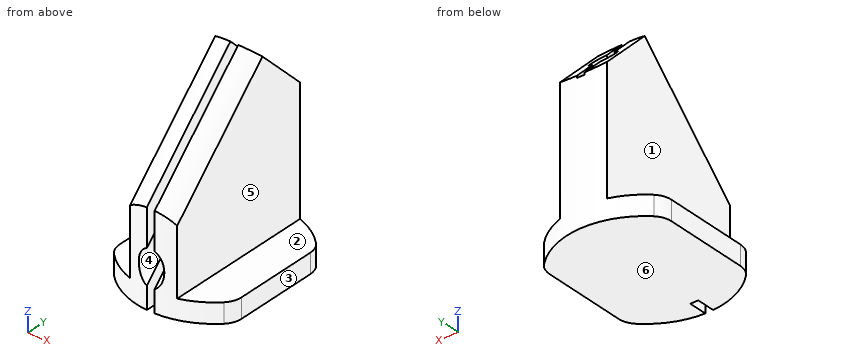
from build123d import *

# Parameters (mm, degrees)
BOSS_EXTRUDE1_DEPTH     = 50
CUT_EXTRUDE2_DEPTH      = 21
CUT_EXTRUDE2_DEPTH_BACK = 21
CUT_EXTRUDE3_DEPTH      = 10.5
CUT_EXTRUDE3_DEPTH_BACK = 22.5
CUT_EXTRUDE4_DEPTH      = 54.639610307


with BuildPart() as part:
    # Sketch1 → Boss-Extrude1 (new body)
    with BuildSketch(Plane.XY):
        with BuildLine():
            Line((-15.5, 10.712142643), (-15.5, -10.712142643))
            ThreePointArc((-15.5, -10.712142643), (-15.109772229, -12.648634316), (-14, -14.282856857))
            ThreePointArc((-14, -14.282856857), (0, -20), (14, -14.282856857))
            ThreePointArc((14, -14.282856857), (15.109772229, -12.648634316), (15.5, -10.712142643))
            Line((15.5, -10.712142643), (15.5, 10.712142643))
            ThreePointArc((15.5, 10.712142643), (15.109772229, 12.648634316), (14, 14.282856857))
            ThreePointArc((14, 14.282856857), (0, 20), (-14, 14.282856857))
            ThreePointArc((-14, 14.282856857), (-15.109772229, 12.648634316), (-15.5, 10.712142643))
        make_face()
    extrude(amount=BOSS_EXTRUDE1_DEPTH)

    # Sketch3 → Cut-Extrude2 (cut, two sides)
    with BuildSketch(Plane(origin=(0, 0, 0), x_dir=(1, 0, 0), z_dir=(0, 1, 0))) as cut_extrude2_sk:
        Polygon((-142.514750581, -5), (-18.067603989, -5), (-6, -5), (-6, -53.756778028), (6, -53.756778028), (6, -5), (19.848795464, -5), (144.295942056, -5), (144.295942056, -253.894293184), (-142.514750581, -253.894293184), align=None)
    extrude(amount=CUT_EXTRUDE2_DEPTH, mode=Mode.SUBTRACT)
    extrude(cut_extrude2_sk.sketch, amount=-CUT_EXTRUDE2_DEPTH_BACK, mode=Mode.SUBTRACT)

    # Sketch4 → Cut-Extrude3 (cut, two sides)
    with BuildSketch(Plane.ZY.offset(6)) as cut_extrude3_sk:
        Polygon((143.928068638, -88.070204261), (54.263494486, 1.594369891), (31.585867619, 24.271996758), (-58.078706533, 113.93657091), (121.250441771, 293.265719213), (323.257216942, 91.258944042), align=None)
    extrude(amount=CUT_EXTRUDE3_DEPTH, mode=Mode.SUBTRACT)
    extrude(cut_extrude3_sk.sketch, amount=-CUT_EXTRUDE3_DEPTH_BACK, mode=Mode.SUBTRACT)

    # Sketch5 → Cut-Extrude4 (cut, through all)
    with BuildSketch(Plane(origin=(0, 27.928932188, 27.928932188), x_dir=(1, 0, 0), z_dir=(0, 0.707106781, 0.707106781))):
        with BuildLine():
            Line((-7.514532889, -27.552153908), (-7.514532889, -51.5106924))
            Line((-7.514532889, -51.5106924), (9.293928827, -51.5106924))
            Line((9.293928827, -51.5106924), (9.293928827, -24.418415532))
            ThreePointArc((9.293928827, -24.418415532), (6.107254228, -28.917224685), (1, -30.993310676))
            Line((1, -30.993310676), (1, -24.305532655))
            ThreePointArc((1, -24.305532655), (3.25, -21.213203436), (1, -18.120874216))
            Line((1, -18.120874216), (1, -10.845979058))
            Line((1, -10.845979058), (-1, -10.845979058))
            Line((-1, -10.845979058), (-1, -18.120874216))
            ThreePointArc((-1, -18.120874216), (-3.25, -21.213203436), (-1, -24.305532655))
            Line((-1, -24.305532655), (-1, -30.993310676))
            ThreePointArc((-1, -30.993310676), (-4.591808745, -29.906062003), (-7.514532889, -27.552153908))
        make_face()
    extrude(amount=-CUT_EXTRUDE4_DEPTH, mode=Mode.SUBTRACT)


solid = part.part
Work out the finished part from the listing and answer in its coordinate system (mm). Face numbers are marked on the shaded views. A direction names the side the tool comes from. Give positions to 0.01 mm unless a question says otherwise; leave off trailing zeros. Loops run counter-clockwise (first coordinate to the right, second up) from the corner with the lowest first, then second, coordinate; pieces in that order, holes last. Notation, with made-up numbers: (-35.75, 14) - (-19.75, 14) arc R35 cw to (-19.75, 49) - close; hole circle Ø11 at (2, 80). An arc over 180 degrees is marked (long way). Answer in a Markdown table with one row per item. Add a question column.
Q1. The part is cut by section A-A (x = -2.5). Determine the outline of the cut face in (y, z).
Q2. The part is cut by section D-D (x = 4). Determine the outline of the cut face in (y, z), and give its area (3 significant figures).
Q3. Consider line 1 along X through (y, z) = (6, 29.5); line 2 along Z through (x, y) = (-8, -9); line 3 along X through (y, z) = (12, 13). Determine where each line is inside the solid, lowest interval first.
Q4. A tool of negligible diameter and unlimited length cuts with its end or side. For the marked faces 1, 2 and 3, from which of +Z, -Z, +X, -X, +Y, -Y can it reach the whole face along a straight path? Write none if from no direction.
Q5. Determine the mould class of the marked faces 4, 5 and 6 for opening direction X: released by +X, released by -X, zero draft, split by the parting line, or undercut.
Q6. Each of these flat-tipped pins is pushed along its axis until it touches: P1, Ø12, axis at x = -9, z = 22.5, coming from the +Y side; P2, Ø5, axis at x = -9, y = 1.5, coming from the +Z side; P3, Ø15.5, axis at y = -11.5, z = 34, coming from the +X side. Where does it stop, or does it pass through?
Q7. The part is cut by section B-B (x = 12). Determine the outline of the cut face in (y, z).
Q8. The part is cut by section C-C (x = -9). Determine the outline of the cut face in (y, z), and give its area (3 significant figures).
Solution:
| question | item | result |
|---|---|---|
| 1 | outline | (-19.84, 0) - (19.84, 0) - (19.84, 36.01) - (14.4, 41.46) - (-19.84, 7.22) - close; (-19.84, 13.09) - (11.46, 44.4) - (6.21, 49.65) - (-19.84, 23.6) - close |
| 2 | outline | (-19.6, 0) - (19.6, 0) - (19.6, 36.26) - (6.58, 49.28) - (-19.6, 23.1) - close |
| 2 | area | 1,500 mm² |
| 3 | line 1 | x = -6 to -1, 1 to 6 |
| 3 | line 2 | z = 0 to 5 |
| 3 | line 3 | x = -6 to 6 |
| 4 | face 1 | +Z, -X, +Y, -Y |
| 4 | face 2 | +Z, +X, +Y, -Y |
| 4 | face 3 | +Z, -Z, +X, +Y, -Y |
| 5 | face 4 | undercut |
| 5 | face 5 | released by +X |
| 5 | face 6 | zero draft |
| 6 | P1 | stops at y = 19.77 |
| 6 | P2 | stops at z = 5 |
| 6 | P3 | stops at x = 6 |
| 7 | outline | (-16, 0) - (16, 0) - (16, 5) - (-16, 5) - close |
| 8 | outline | (-17.86, 0) - (17.86, 0) - (17.86, 5) - (-17.86, 5) - close |
| 8 | area | 179 mm² |
